from build123d import *

# Parameters (mm, degrees)
BOSS_EXTRUDE2_DEPTH = 3


with BuildPart() as part:
    # Sketch1 → Boss-Extrude2 (new body)
    with BuildSketch(Plane(origin=(0, 0, 0), x_dir=(1, 0, 0), z_dir=(0, 1, 0))):
        with BuildLine():
            Line((83.639689367, 6.764475065), (35.667186692, -8.49628906))
            ThreePointArc((35.667186692, -8.49628906), (32.821791297, -9.165503452), (29.907418735, -9.39034879))
            Line((29.907418735, -9.39034879), (13.331621464, -9.39034879))
            ThreePointArc((13.331621464, -9.39034879), (11.831621464, -10.89034879), (13.331621464, -12.39034879))
            Line((13.331621464, -12.39034879), (31.335553361, -12.39034879))
            ThreePointArc((31.335553361, -12.39034879), (32.706920816, -23.000925987), (31.335553361, -33.611503185))
            Line((31.335553361, -33.611503185), (5.672878156, -30.687610674))
            ThreePointArc((5.672878156, -30.687610674), (4.012715552, -32.008163637), (5.333268515, -33.668326241))
            Line((5.333268515, -33.668326241), (32.258758745, -36.73609835))
            ThreePointArc((32.258758745, -36.73609835), (30.141236011, -40.825580171), (25.83833159, -42.466548678))
            Line((25.83833159, -42.466548678), (3.931607644, -43.234741077))
            Line((3.931607644, -43.234741077), (1.645004408, -44.879459267))
            ThreePointArc((1.645004408, -44.879459267), (-0.44755249, -45.424610965), (-2.363050322, -44.421190413))
            ThreePointArc((-2.363050322, -44.421190413), (-16.657617756, -35.649988568), (-33.406545395, -36.511419261))
            ThreePointArc((-33.406545395, -36.511419261), (-35.065515769, -36.818007167), (-36.732015424, -36.555409102))
            Line((-36.732015424, -36.555409102), (-43.072013441, -34.41346595))
            ThreePointArc((-43.072013441, -34.41346595), (-44.756883472, -34.602804193), (-45.690953078, -36.017777677))
            ThreePointArc((-45.690953078, -36.017777677), (-44.377060251, -43.944176391), (-38.701961301, -49.631650596))
            ThreePointArc((-38.701961301, -49.631650596), (-48.89375638, -45.294039559), (-53.199015105, -35.088535957))
            ThreePointArc((-53.199015105, -35.088535957), (-57.963880411, -31.924307539), (-60.880420097, -27.003933658))
            ThreePointArc((-60.880420097, -27.003933658), (-60.719986784, -25.061085947), (-59.232742508, -23.80072864))
            ThreePointArc((-59.232742508, -23.80072864), (-56.720776297, -23.205324241), (-54.14697512, -23.005253893))
            ThreePointArc((-54.14697512, -23.005253893), (-52.817288904, -22.454479829), (-52.26651484, -21.124793613))
            Line((-52.26651484, -21.124793613), (-52.26651484, -18.255253893))
            ThreePointArc((-52.26651484, -18.255253893), (-51.768596368, -17.053172365), (-50.56651484, -16.555253893))
            Line((-50.56651484, -16.555253893), (-50.18504008, -16.555253893))
            Line((-50.18504008, -16.555253893), (-50.18504008, -21.008976099))
            ThreePointArc((-50.18504008, -21.008976099), (-49.292805972, -23.163019785), (-47.138762286, -24.055253893))
            Line((-47.138762286, -24.055253893), (-38.258057554, -24.055253893))
            ThreePointArc((-38.258057554, -24.055253893), (-32.429820226, -23.139270307), (-27.163537606, -20.479638066))
            Line((-27.163537606, -20.479638066), (-18.213895237, -14.042299326))
            ThreePointArc((-18.213895237, -14.042299326), (-17.803794916, -13.348327859), (-18.036830501, -12.576658832))
            ThreePointArc((-18.036830501, -12.576658832), (-21.621060958, -9.471725354), (-25.963310125, -7.565894288))
            Line((-25.963310125, -7.565894288), (-55.30954126, 0.349304832))
            ThreePointArc((-55.30954126, 0.349304832), (-56.903028243, 0.142191478), (-57.883342437, -1.131025232))
            Line((-57.883342437, -1.131025232), (-57.883342437, -6.467193959))
            Line((-57.883342437, -6.467193959), (-59.970418868, -6.467193959))
            ThreePointArc((-59.970418868, -6.467193959), (-62.745333472, -5.626502668), (-64.58710946, -3.387133535))
            ThreePointArc((-64.58710946, -3.387133535), (-65.510981808, 5.487804074), (-61.413967112, 13.414501258))
            ThreePointArc((-61.413967112, 13.414501258), (-58.998069827, 14.801189981), (-56.215124926, 14.680016601))
            Line((-56.215124926, 14.680016601), (-8.465601761, -1.451970173))
            Line((-8.465601761, -1.451970173), (-8.465601761, -6.951970173))
            ThreePointArc((-8.465601761, -6.951970173), (-6.965601761, -8.451970173), (-5.465601761, -6.951970173))
            Line((-5.465601761, -6.951970173), (-5.465601761, 12.336199013))
            Line((-5.465601761, 12.336199013), (3.240530108, 9.661679805))
            add(Edge.make_bspline(
                [(3.240530108, 9.661679805), (13.894797432, -11.003486244), (52.167573777, 8.728675087), (90.440350123, 28.460836418), (79.7860828, 49.126002466)],
                knots=[0, 0, 0, 1.570796327, 1.570796327, 3.141592654, 3.141592654, 3.141592654], degree=2, weights=[1, 0.707106781, 1, 0.707106781, 1]))
            ThreePointArc((79.7860828, 49.126002466), (80.072864648, 50.032062802), (80.980537261, 49.750425469))
            ThreePointArc((80.980537261, 49.750425469), (84.258913327, 36.128474368), (80.573020022, 22.611096962))
            ThreePointArc((80.573020022, 22.611096962), (80.977131886, 20.56443692), (83.060820169, 20.666254716))
            ThreePointArc((83.060820169, 20.666254716), (96.799731472, 40.865743936), (100.995247842, 64.931792447))
            ThreePointArc((100.995247842, 64.931792447), (102.023911204, 66.097176073), (103.234366802, 65.121950687))
            ThreePointArc((103.234366802, 65.121950687), (102.922479327, 43.686615501), (96.524889391, 23.225879655))
            ThreePointArc((96.524889391, 23.225879655), (96.918331366, 21.131130375), (99.034577715, 20.877610113))
            ThreePointArc((99.034577715, 20.877610113), (110.533106389, 30.92010294), (117.098161764, 44.70298623))
            ThreePointArc((117.098161764, 44.70298623), (118.133339849, 45.419031095), (118.968319872, 44.477159407))
            ThreePointArc((118.968319872, 44.477159407), (109.792721336, 19.953626833), (86.773007072, 7.476126539))
            ThreePointArc((86.773007072, 7.476126539), (85.19127768, 7.186654615), (83.639689367, 6.764475065))
        make_face()
    extrude(amount=BOSS_EXTRUDE2_DEPTH)


solid = part.part
Geometry: final body of the model. Coordinates: model frame, mm. A direction names the side the tool comes from. Coordinates: 2 decimals unless noted, no trailing zeros. Order: outer loops, then holes, each group sorted by start corner. A loop starts at its lowest first (then second) coordinate and runs counter-clockwise, first axis right, second up.
(1) Access query for faces 1 (the face through (-44.43, 1.48, 43.84)), 2 (the face through (-21.56, 1.48, 9.51)), 3 (the face through (59.99, 1.48, 0.76)). Directions: +Z, -Z, +X, -X, +Y, -Y. A direction counts if a zero-diameter tool reaches every point of the face in a straight line with its end or side. Return the directions, or none.
(2) Material intervals for probe 1 along Z at (x, y) = (16, 2.7); probe 2 along Z at (x, y) = (23, 1.1); probe 3 along X at (y, z) = (2.05, -21), sorted ascending.
(3) Section query A-A (x = -24). Return the cut outline in (y, z).
(4) Draft query along Z for faces 4 (the face through (-32.675, 1.479, -6.727)), 5 (the face through (110.403, 1.479, -30.749)), 6 (the face through (-57.91, 1.48, 31.98)). Return one class per face: pulls with the +Z half, pulls with the -Z half, needs draft (parallel to the pull), parting line crosses it, or undercut.
(5) First-contact query: pin 1 (1.5 mm diameter, centred on y = 2, z = 0.5, fed in from -X); pin 2 (1.5 mm diameter, centred on x = -41, y = 2, fed in from -Z); pin 3 (0.9 mm diameter, centred on y = 2, z = 20.5, fed in from -X); pin 4 (10 mm diameter, centred on x = 72, z = -47.5, fed in from -Y). Flat tips, straight axial feed; report the tip coordinate or a pass-through.
(6) Section query D-D (x = 108). Return the cut outline in (y, z).
(7) Section query B-B (x = 19). State how many separate pieces and enclosed holes the cut face has, plus the area to 3 significant figures.
(8) Section query C-C (z = -59). Return the cut outline in (x, y).
Solution:
1. face 1: +Y, -Y
1. face 2: -X, +Y, -Y
1. face 3: +Z, +X, +Y, -Y
2. probe 1: z = -1.43 to 9.39, 12.39 to 31.86, 34.88 to 42.81
2. probe 2: z = -0.82 to 9.39, 12.39 to 32.66, 35.68 to 42.57
2. probe 3: x = 69.5 to 80.59, 83.41 to 97.08, 99.25 to 110.67
3. outline: (0, -3.8) - (3, -3.8) - (3, 8.24) - (0, 8.24) - close; (0, 18.2) - (3, 18.2) - (3, 34.78) - (0, 34.78) - close
4. face 4: pulls with the -Z half
4. face 5: undercut
4. face 6: pulls with the +Z half
5. pin 1: stops at x = -65.6
5. pin 2: stops at z = -9.79
5. pin 3: stops at x = -52.27
5. pin 4: passes through
6. outline: (0, -27.92) - (3, -27.92) - (3, -18.03) - (0, -18.03) - close
7. separate pieces: 3
7. enclosed holes: 0
7. area: 113 mm2
8. outline: (100.93, 0) - (103.78, 0) - (103.78, 3) - (100.93, 3) - close
